from build123d import *

# Parameters (mm, degrees)
SKETCH1_R           = 2.425
BOSS_EXTRUDE1_DEPTH = 60
SKETCH2_R           = 1.375
CUT_EXTRUDE1_DEPTH  = 11
CUT_EXTRUDE2_START  = -49
SKETCH2_2_R         = 1.375
CUT_EXTRUDE2_DEPTH  = 11


with BuildPart() as part:
    # Sketch1 → Boss-Extrude1 (new body)
    with BuildSketch(Plane(origin=(0, 0, 0), x_dir=(1, 0, 0), z_dir=(0, 1, 0))):
        with Locations(Location((0, 0, 0), (0, 0, 270))):
            Circle(SKETCH1_R)
    extrude(amount=BOSS_EXTRUDE1_DEPTH)

    # Sketch2 → Cut-Extrude1 (cut)
    with BuildSketch(Plane(origin=(0, 60, 0), x_dir=(1, 0, 0), z_dir=(0, 1, 0))):
        with Locations(Location((0, 0, 0), (0, 0, 270))):
            Circle(SKETCH2_R)
    extrude(amount=-CUT_EXTRUDE1_DEPTH, mode=Mode.SUBTRACT)

    # Sketch2<2> → Cut-Extrude2 (cut)
    with BuildSketch(Plane(origin=(0, 60, 0), x_dir=(1, 0, 0), z_dir=(0, 1, 0)).offset(CUT_EXTRUDE2_START)):
        with Locations(Location((0, 0, 0), (0, 0, 270))):
            Circle(SKETCH2_2_R)
    extrude(amount=-CUT_EXTRUDE2_DEPTH, mode=Mode.SUBTRACT)


solid = part.part
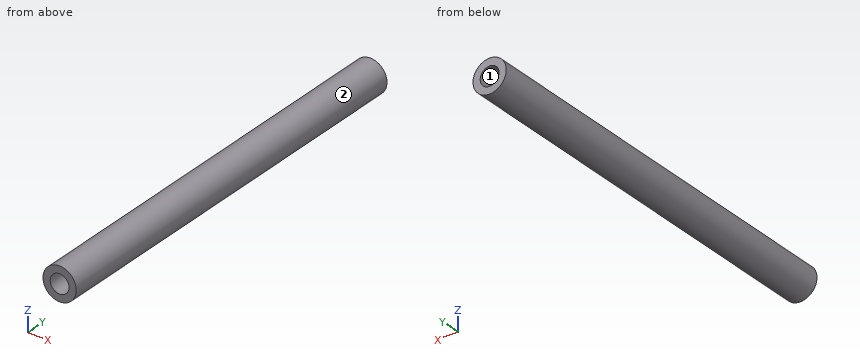
Could you check a few things on this model? Use its own coordinates, in mm. Face numbers are marked on the shaded views. Round coordinates to 2 decimals unless told otherwise and drop trailing zeros. Order: outer loops, then holes, each group sorted by start corner. A loop starts at its lowest first (then second) coordinate and runs counter-clockwise, first axis right, second up.
Q1. Please list where these lines run through material, in increasing order: probe 1 along X at (y, z) = (53.5, 0) (3 decimals); probe 2 along X at (y, z) = (34, 0.1); probe 3 along Y at (x, z) = (0.95, -0.75).
Geometry says:
probe 1: x = -2.425 to -1.375, 1.375 to 2.425
probe 2: x = -2.42 to 2.42
probe 3: y = 11 to 49
Q2. Imagine slicing it at A-A, the plane z = 0. List the corners of the cut face in (x, y) for me (3 decimals).
Geometry says:
outline: (-2.425, 0) - (-1.375, 0) - (-1.375, 11) - (1.375, 11) - (1.375, 0) - (2.425, 0) - (2.425, 60) - (1.375, 60) - (1.375, 49) - (-1.375, 49) - (-1.375, 60) - (-2.425, 60) - close
Q3. Thinking about a two-plate mould opening in Z: for the marked faces 1 and 2, which applies, released by +Z, released by -Z, zero draft, split by the parting line, or undercut?
Geometry says:
face 1: undercut
face 2: split by the parting line
Q4. I'm going to push flat-ended pins straight in: P1, Ø2, axis at x = 0, z = 0, coming from the -Y side; P2, Ø0.8, axis at x = -0.5, z = -0.5, coming from the +Y side. Where does each tip first touch, or does it pass through?
Geometry says:
P1: stops at y = 11
P2: stops at y = 49
Q5. Imagine slicing it at B-B, the plane x = 0. List the corners of the cut face in (y, z) for me (3 decimals), then the cut area to 4 significant figures.
Geometry says:
outline: (0, -2.425) - (60, -2.425) - (60, -1.375) - (49, -1.375) - (49, 1.375) - (60, 1.375) - (60, 2.425) - (0, 2.425) - (0, 1.375) - (11, 1.375) - (11, -1.375) - (0, -1.375) - close
area: 230.5 mm2
Q6. Imagine slicing it at C-C, the plane y = 53.5. List the corners of the cut face in (x, z) for me (3 decimals).
Geometry says:
outline: circle Ø4.85 at (0, 0); hole circle Ø2.75 at (0, 0)
Q7. Imagine slicing it at D-D, the plane y = 20.5. List the corners of the cut face in (x, z) for me (3 decimals).
Geometry says:
outline: circle Ø4.85 at (0, 0)
